Read the model definition and answer for the solid it produces. Units are mm, in the model's axes. A direction names the side the tool comes from. Round coordinates to 2 decimals unless told otherwise and drop trailing zeros. Order: outer loops, then holes, each group sorted by start corner. A loop starts at its lowest first (then second) coordinate and runs counter-clockwise, first axis right, second up. Notation, with made-up numbers: (67.5, 21) - (110.5, 21) arc R8 ccw to (110.5, 35) - close; hole circle Ø1 at (65.25, 43). An arc over 180 degrees is marked (long way). Put each result on its own line as item: value. Start each with the question number.
Q1. Find the intervals of material crossed by line 1 along Z through (x, y) = (20.25, 0.25); line 2 along X through (y, z) = (-0.75, 3.25); line 3 along X through (y, z) = (5, 2), in increasing order. Write a range as from..to.
Q2. This flat-tipped pin is pushed along its axis until it touches: pin 1 Ø1.5 at (x, z) = (22.5, 3.5) entering from +Y. Where does it stop, or does it pass through?
Q3. For a pull along X with two mould halves and no side action, classify faces 4 (the face through (6.072, 1.399, 6.899)), 5 (the face through (15, 1, 2)), 6 (the face through (15.61, 5.06, 0.29)), 7 (the face through (23.35, -2.33, 2.17)) as pulls with the +X half, pulls with the -X half, needs draft (parallel to the pull), parting line crosses it, or undercut.
Q4. Section B-B on z = 3.75 is taken. Give the vertices of the cut face in (x, y), then the cut area to 3 significant figures.
Q5. Section C-C on y = -1 is taken. Give the vertices of the cut face in (x, z), then the cut area to 3 significant figures.
Q6. Section A-A on x = 13.75 is taken. Give the vertices of the cut face in (y, z), then the cut area to 3 significant figures.
Q7. Which of the six approach directions +Z, -Z, +X, -X, +Y, -Y give full straight-line access (tool end or side, diameter ignored) to faces 1 (the face through (7.67, -2.33, 2.15)), 2 (the face through (7.66, 5.06, 2.14)), 3 (the face through (23.216, 1.406, 5.199))?
from build123d import *

# Parameters (mm, degrees)
F0_W     = 20
F0_H     = 8
F1_DEPTH = 7.5
F2_T     = -2
F3_DEPTH = 25
F4_R     = 2
F5_R     = 1
F6_R     = 1
F7_SIZE  = 0.5
F9_DEPTH = 1


with BuildPart() as f1:
    # F0 (on Top) → F1 (new body)
    with BuildSketch(Plane.XY):
        with Locations((15.5013518035, 1.3572655581)):
            Rectangle(F0_W, F0_H)
    extrude(amount=F1_DEPTH)

    # F2
    f2_openings = [f1.faces().sort_by_distance(p)[0] for p in [
        (15.501352, -2.642734, 3.75),
    ]]
    offset(amount=F2_T, openings=f2_openings)

    # F3 (cut): a face of the model
    f3_faces = [f1.faces().sort_by_distance(p)[0] for p in [
        (15.5013518035, 3.3572655581, 3.75),
    ]]
    extrude(f3_faces, amount=-F3_DEPTH, mode=Mode.SUBTRACT)

    # F4
    f4_edges = [f1.edges().sort_by_distance(p)[0] for p in [
        (25.501352, 1.357266, 7.5),
        (25.501352, 1.357266, 0),
        (5.501352, 1.357266, 7.5),
        (5.501352, 1.357266, 0),
    ]]
    fillet(f4_edges, radius=F4_R)

    # F5
    f5_edges = [f1.edges().sort_by_distance(p)[0] for p in [
        (7.501352, 1.357266, 5.5),
        (7.501352, 1.357266, 2),
        (23.501352, 1.357266, 5.5),
        (23.501352, 1.357266, 2),
    ]]
    fillet(f5_edges, radius=F5_R)

    # F6
    f6_edges = [f1.edges().sort_by_distance(p)[0] for p in [
        (15.501352, -2.642734, 0),
        (15.501352, 5.357266, 0),
    ]]
    fillet(f6_edges, radius=F6_R)

    # F7
    f7_edges = [f1.edges().sort_by_distance(p)[0] for p in [
        (15.501352, -2.642734, 5.5),
        (15.501352, 5.357266, 5.5),
    ]]
    chamfer(f7_edges, length=F7_SIZE)

    # F8 (on face) → F9 (join)
    with BuildSketch(Plane.XY.offset(7.5)):
        Polygon((9.5939766616, 4.3572655581), (8.2856733352, 4.3572655581), (8.2856733352, -1.6427344419), (9.5939766616, -1.6427344419), (9.5939766616, 1.0383471381), (10.6051471084, -1.6427344419), (12.1620288119, -1.6427344419), (10.7613857836, 1.5246823896), (12.1620288119, 4.3572655581), (10.5070443824, 4.3572655581), (9.5939766616, 2.1014690865), align=None)
        Polygon((16.4463743567, 4.3572655581), (12.1620288119, 4.3572655581), (12.1620288119, -1.6427344419), (16.4463743567, -1.6427344419), (16.4463743567, 1.214308897), (14.3119534478, 1.214308897), (14.3119534478, 0.6480877637), (15.4404239729, 0.6480877637), (15.4404239729, 0), (13.5471438989, 0), (13.5471438989, 3.0533354729), (15.4435969889, 3.0533354729), (15.4435969889, 2.0766169764), (16.4463743567, 2.0766169764), align=None)
    extrude(amount=-F9_DEPTH)


solid = f1.part
Findings:
1. line 1: 0..2, 5.5..7.5
1. line 2: 5.5..7.5, 23.5..25.5
1. line 3: 5.74..7.95, 23.05..25.27
2. pin 1: through
3. face 4: pulls with the -X half
3. face 5: undercut
3. face 6: needs draft
3. face 7: undercut
4. outline: (5.5, -1.64) arc R1 ccw to (6.5, -2.64) - (7, -2.64) - (7.5, -2.14) - (7.5, 4.86) - (7, 5.36) - (6.5, 5.36) arc R1 ccw to (5.5, 4.36) - close; (23.5, -2.14) - (24, -2.64) - (24.5, -2.64) arc R1 ccw to (25.5, -1.64) - (25.5, 4.36) arc R1 ccw to (24.5, 5.36) - (24, 5.36) - (23.5, 4.86) - close
4. area: 30.6 mm2
5. outline: (5.5, 2) arc R2 ccw to (7.5, 0) - (23.5, 0) arc R2 ccw to (25.5, 2) - (25.5, 5.5) arc R2 ccw to (23.5, 7.5) - (7.5, 7.5) arc R2 ccw to (5.5, 5.5) - close; hole (7.5, 3) arc R1 ccw to (8.5, 2) - (22.5, 2) arc R1 ccw to (23.5, 3) - (23.5, 4.5) arc R1 ccw to (22.5, 5.5) - (8.5, 5.5) arc R1 ccw to (7.5, 4.5) - close
5. area: 91.4 mm2
6. outline: (-2.64, 1) arc R1 ccw to (-1.64, 0) - (4.36, 0) arc R1 ccw to (5.36, 1) - (5.36, 1.5) - (4.86, 2) - (-2.14, 2) - (-2.64, 1.5) - close; (-2.64, 6) - (-2.14, 5.5) - (4.86, 5.5) - (5.36, 6) - (5.36, 6.5) arc R1 ccw to (4.36, 7.5) - (-1.64, 7.5) arc R1 ccw to (-2.64, 6.5) - close
6. area: 30.6 mm2
7. face 1: -Y
7. face 2: +Y
7. face 3: +Y, -Y
